Here's how the part is built. I have some questions about the finished solid (model axes, mm). A direction names the side the tool comes from. Give positions to 0.01 mm unless a question says otherwise; leave off trailing zeros. Write each loop counter-clockwise with the first axis right and the second up, starting at its lowest first coordinate (ties: lowest second). Pieces come first, ordered by that corner, then holes. Notation, with made-up numbers: (-25.5, 3.25) -> (2.5, 3.25) arc R26 cw to (2.5, 19.25) -> close; hole circle Ø2 at (4, -15). An arc over 180 degrees is marked (long way). Answer as CSV lines item,"result". Start each with the question number.
from build123d import *

# Parameters (mm, degrees)
F1_DEPTH = 1.075
F2_W     = 20.9250352345
F2_H     = 5.8195129968
F2_R     = 0.5
F3_DEPTH = 12.5
F4_R     = 0.5
F5_DEPTH = 12.5


# Not quite as in the source:
# - ends of sketch curves that miss each other by under 0.0002 mm in the source are joined


with BuildPart() as f1:
    # F0 (on Front) → F1 (new body, symmetric)
    with BuildSketch(Plane.XZ):
        with BuildLine():
            Line((0, 0.5), (0, 0))
            Line((0, 0), (14.5, 0))
            ThreePointArc((14.5, 0), (14.6687831398, -0.051983364), (14.7790735103, -0.1899183219))
            Line((14.7790735103, -0.1899183219), (15, -0.75))
            Line((15, -0.75), (15.645704163, -0.55329938))
            ThreePointArc((15.645704163, -0.55329938), (15.8994973246, -0.3756690667), (15.9999418448, -0.082625733))
            Line((15.9999418448, -0.082625733), (16, -0.075))
            Line((16, -0.075), (18, -0.075))
            Line((18, -0.075), (18, 0.825))
            Line((18, 0.825), (15.9683748499, 0.825))
            ThreePointArc((15.9683748499, 0.825), (15.7850438563, 0.5892080819), (15.5, 0.5))
            Line((15.5, 0.5), (6.35, 0.5))
            ThreePointArc((6.35, 0.5), (5.7666369055, 0.7416369055), (5.525, 1.325))
            ThreePointArc((5.525, 1.325), (5.4508825364, 1.7619415066), (5.2368220677, 2.15))
            Line((5.2368220677, 2.15), (4.2, 2.15))
            ThreePointArc((4.2, 2.15), (5.025, 1.325), (4.2, 0.5))
            Line((4.2, 0.5), (0, 0.5))
        make_face()
        with BuildLine():
            Line((0, 2.15), (4.2, 2.15))
            Line((4.2, 2.15), (5.2368220677, 2.15))
            ThreePointArc((5.2368220677, 2.15), (4.7755432217, 2.5184718262), (4.2, 2.65))
            Line((4.2, 2.65), (0, 2.65))
            Line((0, 2.65), (0, 2.15))
        make_face()
    extrude(amount=F1_DEPTH, both=True)

    # F2 (on Top) → F3 (cut, symmetric)
    with BuildSketch(Plane.XY):
        with Locations((8.4883153904, -0.0547866803)):
            Rectangle(F2_W, F2_H)
        with BuildLine():
            Line((6, 1.075), (17.1671358116, 0.8498272554))
            ThreePointArc((17.1671358116, 0.8498272554), (17.7570689581, 0.5949514939), (18, 0))
            ThreePointArc((18, 0), (17.7570689581, -0.5949514939), (17.1671358116, -0.8498272554))
            Line((17.1671358116, -0.8498272554), (6, -1.075))
            Line((6, -1.075), (1.075, -1.075))
            ThreePointArc((1.075, -1.075), (0.3148602102, -0.7601397898), (0, 0))
            ThreePointArc((0, 0), (0.3148602102, 0.7601397898), (1.075, 1.075))
            Line((1.075, 1.075), (6, 1.075))
        make_face(mode=Mode.SUBTRACT)
        with Locations((1.075, 0)):
            Circle(F2_R)
        with Locations((3.075, 0)):
            Circle(F2_R)
    extrude(amount=F3_DEPTH, both=True, mode=Mode.SUBTRACT)

    # F4 (on Top) → F5 (cut, symmetric)
    with BuildSketch(Plane.XY):
        with Locations((17.15, 0)):
            Circle(F4_R)
    extrude(amount=F5_DEPTH, both=True, mode=Mode.SUBTRACT)


solid = f1.part
Item 1: If we section it at D-D (x = 9): Please give me the cut outline in (y, z).
Item 2: For faces 4 (the face through (16.5, -0.2, -0.075)), 5 (the face through (1.537, -0.192, 0.246)), 6 (the face through (5.77, -0.02, 0.74)), 7 (the face through (16.5, -0.2, 0.825)), which set-ups out of +Z, -Z, +X, -X, +Y, -Y let a thin tool reach every point of the face, with its end or its side?
Item 3: We'd pull the mould along Z, two halves only. Please class faces 1 (the face through (3.5, 1.075, 0.2)), 2 (the face through (2, 0, 0.5)), 3 (the face through (7, 0, 0)): released by +Z, released by -Z, zero draft, split by the parting line, or undercut.
Item 4: If I drill on line 1 (Y direction, x = 17.15, z = 0.5); line 2 (Z direction, x = 7, y = -0.55); line 3 (Z direction, x = 16.25, y = -0.3) (3 decimals), over which ranges is the centre line in solid material (lowest first)? Write a range as [from, to].
Item 5: If we section it at A-A (x = 4): Please give me the cut outline in (y, z) (3 decimals), and give its area (3 significant figures).
Item 6: If we section it at C-C (z = 1.5): Please give me the cut outline in (x, y) (3 decimals).
Item 7: I'm going to push flat-ended pins straight in: pin 1 (0.6 mm diameter, centred on x = 1.5, y = 0, fed in from -Z); pin 2 (2 mm diameter, centred on x = 7.5, z = 0, fed in from +Y); pin 3 (1 mm diameter, centred on x = 13, z = 0, fed in from +Y); pin 4 (0.6 mm diameter, centred on x = 1, y = 0, fed in from +Z). Where does each tip first touch, or does it pass through?
Item 8: If we section it at B-B (y = 0): State how many separate pieces and enclosed holes the cut face has, and give its area (3 significant figures).
Final values:
1,outline,"(-1.01, 0) -> (1.01, 0) -> (1.01, 0.5) -> (-1.01, 0.5) -> close"
2,face 4,"-Z, +X, +Y, -Y"
2,face 5,"+Z, -Z"
2,face 6,"+Z, +Y, -Y"
2,face 7,"+Z, +X, +Y, -Y"
3,face 1,"zero draft"
3,face 2,"undercut"
3,face 3,"released by -Z"
4,line 1,"[-0.85, -0.5], [0.5, 0.85]"
4,line 2,"[0, 0.5]"
4,line 3,"[-0.075, 0.825]"
5,outline,"(-1.075, 0) -> (1.075, 0) -> (1.075, 0.5) -> (-1.075, 0.5) -> close; (-1.075, 2.15) -> (1.075, 2.15) -> (1.075, 2.65) -> (-1.075, 2.65) -> close"
5,area,"2.15 mm2"
6,outline,"(5.006, -1.075) -> (5.513, -1.075) -> (5.513, 1.075) -> (5.006, 1.075) -> close"
7,pin 1,"z = 0"
7,pin 2,"y = 1.06"
7,pin 3,"y = 0.94"
7,pin 4,"through"
8,separate pieces,"6"
8,enclosed holes,"0"
8,area,"11.3 mm2"
